Can you work these out from the model? Positions are in its coordinate system, mm. A direction names the side the tool comes from. Coordinates: 2 decimals unless noted, no trailing zeros. Loops run counter-clockwise (first coordinate to the right, second up) from the corner with the lowest first, then second, coordinate; pieces in that order, holes last.
```python
from build123d import *

# Parameters (mm, degrees)
SKETCH1_W           = 25.4
SKETCH1_H           = 38.1
BOSS_EXTRUDE1_DEPTH = 3.175
SKETCH2_R           = 9.525
BOSS_EXTRUDE2_DEPTH = 19.05
SKETCH3_R           = 6.477
CUT_EXTRUDE1_DEPTH  = 32.908355097
SKETCH4_R           = 1.905
CUT_EXTRUDE2_DEPTH  = 30.784140075


with BuildPart() as part:
    # Sketch1 → Boss-Extrude1 (new body)
    with BuildSketch(Plane.XY):
        Rectangle(SKETCH1_W, SKETCH1_H)
    extrude(amount=BOSS_EXTRUDE1_DEPTH)

    # Sketch2 → Boss-Extrude2 (add)
    with BuildSketch(Plane.XY.offset(3.175)):
        with Locations(Location((0, 0, 0), (0, 0, 180))):
            Circle(SKETCH2_R)
    extrude(amount=BOSS_EXTRUDE2_DEPTH)

    # Sketch3 → Cut-Extrude1 (cut, through all)
    with BuildSketch(Plane.XY.offset(22.225)):
        Circle(SKETCH3_R)
    extrude(amount=-CUT_EXTRUDE1_DEPTH, mode=Mode.SUBTRACT)

    # Sketch4 → Cut-Extrude2 (cut, through all)
    with BuildSketch(Plane.XY.offset(3.175)):
        with Locations((0, 12.7)):
            Circle(SKETCH4_R)
        with Locations((0, -12.7)):
            Circle(SKETCH4_R)
    extrude(amount=-CUT_EXTRUDE2_DEPTH, mode=Mode.SUBTRACT)


solid = part.part
```
(1) Which directions (+Z, -Z, +X, -X, +Y, -Y) give clear straight access to the entire face, cutting with the end or side of a thin tool? Please do faces 1 (the flat face through (12.7, 0, 2)), 2 (the cylindrical face through (2.06, 9.3, 12.57)).
Check values:
face 1: +Z, -Z, +X, +Y, -Y
face 2: +Z
(2) I want a section at A-A on x = 0. Write out the boundary of the cut face in (y, z) (3 decimals), then the cut area to 3 significant figures.
Check values:
outline: (-19.05, 0) - (-14.605, 0) - (-14.605, 3.175) - (-19.05, 3.175) - close; (-10.795, 0) - (-6.477, 0) - (-6.477, 22.225) - (-9.525, 22.225) - (-9.525, 3.175) - (-10.795, 3.175) - close; (6.477, 0) - (10.795, 0) - (10.795, 3.175) - (9.525, 3.175) - (9.525, 22.225) - (6.477, 22.225) - close; (14.605, 0) - (19.05, 0) - (19.05, 3.175) - (14.605, 3.175) - close
area: 172 mm2
(3) I'm going to push flat-ended pins straight in: pin 1 (7.5 mm diameter, centred on x = -2, y = 3, fed in from +Z) (3 decimals); pin 2 (6 mm diameter, centred on x = 0, y = -12.7, fed in from +Z) (3 decimals); pin 3 (6 mm diameter, centred on y = 10, z = 16, fed in from -X); pin 4 (4 mm diameter, centred on x = 0, z = 13.5, fed in from -Y) (3 decimals). Where does each tip first touch, or does it pass through?
Check values:
pin 1: stops at z = 22.225
pin 2: stops at z = 3.175
pin 3: stops at x = -6.46
pin 4: stops at y = -9.525
(4) If I drill on probe 1 along Y at (x, z) = (0, 1.4) (3 decimals); probe 2 along Y at (x, z) = (0, 5.75) (3 decimals); probe 3 along Z at (x, y) = (8.5, 6) (3 decimals), over which ranges is the centre line in solid material (lowest first)?
Check values:
probe 1: y = -19.05 to -14.605, -10.795 to -6.477, 6.477 to 10.795, 14.605 to 19.05
probe 2: y = -9.525 to -6.477, 6.477 to 9.525
probe 3: z = 0 to 3.175
(5) I want a section at C-C on z = 17. Write out the boundary of the cut face in (x, y) (3 decimals), then the cut area to 3 significant figures.
Check values:
outline: circle Ø19.05 at (0, 0); hole circle Ø12.954 at (0, 0)
area: 153 mm2
(6) I want a section at B-B on y = 12.7. Write out the boundary of the cut face in (x, z) (3 decimals), then the cut area to 3 significant figures.
Check values:
outline: (-12.7, 0) - (-1.905, 0) - (-1.905, 3.175) - (-12.7, 3.175) - close; (1.905, 0) - (12.7, 0) - (12.7, 3.175) - (1.905, 3.175) - close
area: 68.5 mm2
(7) I want a section at D-D on x = -3.25. Write out the boundary of the cut face in (y, z) (3 decimals).
Check values:
outline: (-19.05, 0) - (-5.603, 0) - (-5.603, 22.225) - (-8.953, 22.225) - (-8.953, 3.175) - (-19.05, 3.175) - close; (5.603, 0) - (19.05, 0) - (19.05, 3.175) - (8.953, 3.175) - (8.953, 22.225) - (5.603, 22.225) - close
(8) If we mould it in two halves opening along Y, with no side actions, what happens to faces 3 (the flat face through (-9, 5, 3.175)), 4 (the cylindrical face through (-0.41, -14.56, 1.61)), 5 (the flat face through (0, 19.05, 2))? For each: released by +Y, released by -Y, zero draft, split by the parting line, or undercut.
Check values:
face 3: zero draft
face 4: undercut
face 5: released by +Y
